```python
from build123d import *

# Parameters (mm, degrees)
SCHIZZO1_W                          = 60
SCHIZZO1_H                          = 80
ESTRUSIONE_ESTRUSIONE1_DEPTH        = 40
TAGLIO_ESTRUSIONE1_REACH            = 84.462
TAGLIO_ESTRUSIONE2_START            = -8
TAGLIO_ESTRUSIONE2_DEPTH            = 9
TAGLIO_ESTRUSIONE3_START            = -23
TAGLIO_ESTRUSIONE3_DEPTH            = 12
TAGLIO_ESTRUSIONE4_START            = -43
TAGLIO_ESTRUSIONE4_DEPTH            = 20
FORO_FILETTATO_M5X0_8_1_D           = 4.2
FORO_FILETTATO_M5X0_8_1_DEPTH       = 12.7381927
FORO_FILETTATO_M5X0_8_1_CSINK_D     = 5.05
FORO_FILETTATO_M5X0_8_1_CSINK_ANGLE = 90
FORO_FILETTATO_M5X0_8_1_TIP         = 1.2618073


with BuildPart() as part:
    # Schizzo1 → Estrusione-Estrusione1 (new body)
    with BuildSketch(Plane(origin=(0, 0, 0), x_dir=(1, 0, 0), z_dir=(0, 1, 0))):
        Rectangle(SCHIZZO1_W, SCHIZZO1_H)
    extrude(amount=ESTRUSIONE_ESTRUSIONE1_DEPTH)

    # Schizzo2 → Taglio-Estrusione1 (cut, up to next)
    with BuildSketch(Plane(origin=(30, 0, 0), x_dir=(0, 0, -1), z_dir=(1, 0, 0)), mode=Mode.PRIVATE) as taglio_estrusione1_sk1:
        with BuildLine():
            Line((-16.5, 40), (16.5, 40))
            ThreePointArc((16.5, 40), (0, 23.5), (-16.5, 40))
        make_face()
    taglio_estrusione1_tool1 = extrude(taglio_estrusione1_sk1.sketch, amount=-TAGLIO_ESTRUSIONE1_REACH, mode=Mode.PRIVATE) & part.part
    add(taglio_estrusione1_tool1.solids().sort_by_distance((30, 32.997183, 0))[0], mode=Mode.SUBTRACT)

    # Schizzo3 → Taglio-Estrusione2 (cut)
    with BuildSketch(Plane(origin=(30, 0, 0), x_dir=(0, 0, -1), z_dir=(1, 0, 0)).offset(TAGLIO_ESTRUSIONE2_START)):
        with BuildLine():
            Line((16.5, 40), (18.5, 40))
            ThreePointArc((18.5, 40), (0, 21.5), (-18.5, 40))
            Line((-18.5, 40), (-16.5, 40))
            ThreePointArc((-16.5, 40), (0, 23.5), (16.5, 40))
        make_face()
    extrude(amount=-TAGLIO_ESTRUSIONE2_DEPTH, mode=Mode.SUBTRACT)

    # Schizzo4 → Taglio-Estrusione3 (cut)
    with BuildSketch(Plane.ZY.offset(30).offset(TAGLIO_ESTRUSIONE3_START)):
        with BuildLine():
            Line((16.5, 40), (18.5, 40))
            ThreePointArc((18.5, 40), (0, 21.5), (-18.5, 40))
            Line((-18.5, 40), (-16.5, 40))
            ThreePointArc((-16.5, 40), (0, 23.5), (16.5, 40))
        make_face()
    extrude(amount=TAGLIO_ESTRUSIONE3_DEPTH, mode=Mode.SUBTRACT)

    # Schizzo5 → Taglio-Estrusione4 (cut)
    with BuildSketch(Plane.ZY.offset(30).offset(TAGLIO_ESTRUSIONE4_START)):
        with BuildLine():
            Line((16.5, 40), (34, 40))
            ThreePointArc((34, 40), (0, 6), (-34, 40))
            Line((-34, 40), (-16.5, 40))
            ThreePointArc((-16.5, 40), (0, 23.5), (16.5, 40))
        make_face()
    extrude(amount=TAGLIO_ESTRUSIONE4_DEPTH, mode=Mode.SUBTRACT)

    # Foro filettato M5x0.8-1
    with Locations(Plane(origin=(-22, 40, -30), x_dir=(0, 0, 1), z_dir=(0, 1, 0))):
        with Locations((0, 0), (0, 45), (60, 0), (60, 45)):
            CounterSinkHole(FORO_FILETTATO_M5X0_8_1_D / 2, FORO_FILETTATO_M5X0_8_1_CSINK_D / 2, depth=FORO_FILETTATO_M5X0_8_1_DEPTH, counter_sink_angle=FORO_FILETTATO_M5X0_8_1_CSINK_ANGLE)
            with Locations((0, 0, -(FORO_FILETTATO_M5X0_8_1_DEPTH + FORO_FILETTATO_M5X0_8_1_TIP / 2))):  # 118° drill point
                Cone(0, FORO_FILETTATO_M5X0_8_1_D / 2, FORO_FILETTATO_M5X0_8_1_TIP, mode=Mode.SUBTRACT)


solid = part.part
```
The model under review builds one solid part; all positions refer to its coordinate system, in mm. A direction names the side the tool comes from. Round coordinates to 2 decimals unless told otherwise and drop trailing zeros. Loops run counter-clockwise (first coordinate to the right, second up) from the corner with the lowest first, then second, coordinate; pieces in that order, holes last.
1) Consider section C-C on z = -15. State the section outline as (x, y) points, then the cut area to 3 significant figures.
Values follow:
outline: (-30, 0) - (30, 0) - (30, 33.13) - (22, 33.13) - (22, 29.17) - (13, 29.17) - (13, 9.49) - (-7, 9.49) - (-7, 29.17) - (-19, 29.17) - (-19, 33.13) - (-30, 33.13) - close
area: 1,430 mm2
2) Consider section D-D on x = 1.5. State the section outline as (y, z) points.
Values follow:
outline: (0, -40) - (40, -40) - (40, -34) arc R34 cw to (40, 34) - (40, 40) - (0, 40) - close
3) Consider section A-A on y = 31. State the section outline as (x, z) points.
Values follow:
outline: (-30, -40) - (30, -40) - (30, -13.83) - (22, -13.83) - (22, -16.16) - (13, -16.16) - (13, -32.79) - (-7, -32.79) - (-7, -16.16) - (-19, -16.16) - (-19, -13.83) - (-30, -13.83) - close; (-30, 13.83) - (-19, 13.83) - (-19, 16.16) - (-7, 16.16) - (-7, 32.79) - (13, 32.79) - (13, 16.16) - (22, 16.16) - (22, 13.83) - (30, 13.83) - (30, 40) - (-30, 40) - close; hole circle Ø4.2 at (-22, -30); hole circle Ø4.2 at (-22, 30); hole circle Ø4.2 at (23, -30); hole circle Ø4.2 at (23, 30)
4) Clearance check with flat-ended pins moving along their axes: P1, Ø3.5, axis at x = 23, z = -30, coming from the +Y side; P2, Ø5.5, axis at y = 32.5, z = -8.5, coming from the +X side; P3, Ø5, axis at x = -22, z = 30, coming from the +Y side (3 decimals). State where each tip first meets the part, or that it passes through.
Values follow:
P1: stops at y = 27.05
P2: passes through
P3: stops at y = 39.975
5) Wall thickness on line 1 along X through (y, z) = (34.75, 30); line 2 along X through (y, z) = (37.5, 22); line 3 along Z through (x, y) = (-22, 31.25): over which ranges is each line inside the solid? List them lowest first.
Values follow:
line 1: x = -30 to -24.1, -19.9 to -7, 13 to 20.9, 25.1 to 30
line 2: x = -30 to -7, 13 to 30
line 3: z = -40 to -32.1, -27.9 to -13.99, 13.99 to 27.9, 32.1 to 40
6) Tool access review of faces 5 (the face through (26.056, 23.504, -0.363)), 6 (the face through (13, 19, 0)): name each direction out of +Z, -Z, +X, -X, +Y, -Y from which nothing blocks a thin tool from reaching the whole face with its end or side.
Values follow:
face 5: +X, -X, +Y
face 6: +Y
7) Consider section B-B on y = 24.5. State the section outline as (x, z) points, then the cut area to 3 significant figures.
Values follow:
outline: (-30, -40) - (30, -40) - (30, -5.66) - (22, -5.66) - (22, -10.1) - (13, -10.1) - (13, -30.26) - (-7, -30.26) - (-7, -10.1) - (-19, -10.1) - (-19, -5.66) - (-30, -5.66) - close; (-30, 5.66) - (-19, 5.66) - (-19, 10.1) - (-7, 10.1) - (-7, 30.26) - (13, 30.26) - (13, 10.1) - (22, 10.1) - (22, 5.66) - (30, 5.66) - (30, 40) - (-30, 40) - close
area: 2,950 mm2
8) The part is to be moulded in two halves that separate along X. For faces 1 (the face through (-24.423, 23.504, -0.363)), 2 (the face through (-30, 20, 1)), 3 (the face through (30, 20, 1)), 4 (the face through (24.419, 33.332, 31.548)), say which applies: pulls with the +X half, pulls with the -X half, needs draft (parallel to the pull), parting line crosses it, or undercut.
Values follow:
face 1: needs draft
face 2: pulls with the -X half
face 3: pulls with the +X half
face 4: undercut
